Here's how the part is built. I have some questions about the finished solid (model axes, mm). Round coordinates to 2 decimals unless told otherwise and drop trailing zeros. Use one line per item in the form item = value. Start each with the question number.
Q1. I'm going to push flat-ended pins straight in: pin 1 Ø2 at (y, z) = (2, -63) entering from -X; pin 2 Ø1.2 at (y, z) = (2.5, 62) entering from -X. Where does each tip first touch, or does it pass through?
Q2. I need wall thicknesses on line 1 along Z through (x, y) = (-8.5, 0.95); line 2 along Z through (x, y) = (-76.5, 1.7); line 3 along X through (y, z) = (1.1, 21.5). Which ranges of each line are inside material? Lowest first, please. Write a range as from..to.
Q3. I want a section at A-A on y = 0.95. State how many separate pieces and enclosed holes the cut face has, and give its area (3 significant figures).
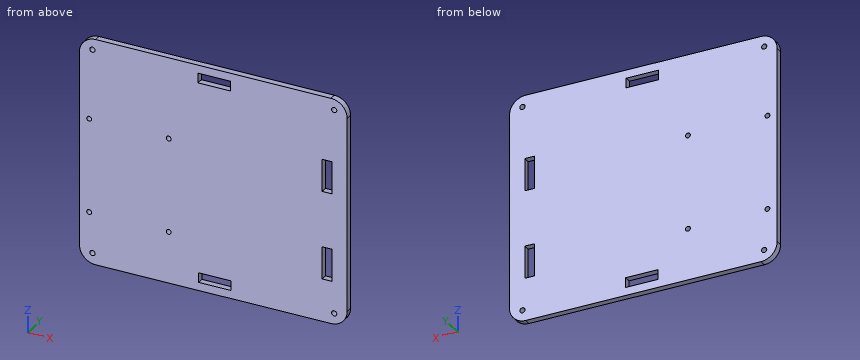
```python
from build123d import *

# Parameters (mm, degrees)
SKETCH1_W           = 165
SKETCH1_H           = 140
BOSS_EXTRUDE1_DEPTH = 4
SKETCH2_R           = 1.6
CUT_EXTRUDE1_DEPTH  = 10
FILLET1_R           = 10
SKETCH3_R           = 1.5
CUT_EXTRUDE2_DEPTH  = 10
SKETCH4_W           = 6
SKETCH4_H           = 20
SKETCH4_W_2         = 20
SKETCH4_H_2         = 6
CUT_EXTRUDE3_DEPTH  = 10


with BuildPart() as part:
    # Sketch1 → Boss-Extrude1 (new body)
    with BuildSketch(Plane(origin=(0, 0, 0), x_dir=(1, 0, 0), z_dir=(0, 1, 0))):
        Rectangle(SKETCH1_W, SKETCH1_H)
    extrude(amount=BOSS_EXTRUDE1_DEPTH)

    # Sketch2 → Cut-Extrude1 (cut)
    with BuildSketch(Plane(origin=(0, 4, 0), x_dir=(1, 0, 0), z_dir=(0, 1, 0))):
        with Locations(Location((-74.5, 63.212121212, 0), (0, 0, 270))):
            Circle(SKETCH2_R)
        with Locations(Location((-74.5, -63.212121212, 0), (0, 0, 270))):
            Circle(SKETCH2_R)
        with Locations(Location((74.5, -63.212121212, 0), (0, 0, 270))):
            Circle(SKETCH2_R)
        with Locations(Location((74.5, 63.212121212, 0), (0, 0, 270))):
            Circle(SKETCH2_R)
    extrude(amount=-CUT_EXTRUDE1_DEPTH, mode=Mode.SUBTRACT)

    # Fillet1
    fillet1_edges = [part.edges().sort_by_distance(p)[0] for p in [
        (82.5, 2, 70),
        (-82.5, 2, 70),
        (-82.5, 2, -70),
        (82.5, 2, -70),
    ]]
    fillet(fillet1_edges, radius=FILLET1_R)

    # Sketch3 → Cut-Extrude2 (cut)
    with BuildSketch(Plane(origin=(0, 4, 0), x_dir=(1, 0, 0), z_dir=(0, 1, 0))):
        with Locations(Location((-76.5, 38.189224362, 0), (0, 0, 270))):
            Circle(SKETCH3_R)
        with Locations(Location((-27.5, 38.189224362, 0), (0, 0, 270))):
            Circle(SKETCH3_R)
        with Locations(Location((-76.5, -19.810775638, 0), (0, 0, 270))):
            Circle(SKETCH3_R)
        with Locations(Location((-27.5, -19.810775638, 0), (0, 0, 270))):
            Circle(SKETCH3_R)
    extrude(amount=-CUT_EXTRUDE2_DEPTH, mode=Mode.SUBTRACT)

    # Sketch4 → Cut-Extrude3 (cut)
    with BuildSketch(Plane(origin=(0, 4, 0), x_dir=(1, 0, 0), z_dir=(0, 1, 0))):
        with Locations((70, 33.680953207)):
            Rectangle(SKETCH4_W, SKETCH4_H)
        with Locations((70, -20.735149517)):
            Rectangle(SKETCH4_W, SKETCH4_H)
        with Locations((0.550060732, -62)):
            Rectangle(SKETCH4_W_2, SKETCH4_H_2)
        with Locations((0.930649546, 62)):
            Rectangle(SKETCH4_W_2, SKETCH4_H_2)
    extrude(amount=-CUT_EXTRUDE3_DEPTH, mode=Mode.SUBTRACT)


solid = part.part
```
Reported:
q1.pin_1 = -82.3
q1.pin_2 = -82.4
q2.line_1 = -70..-65, -59..59, 65..70
q2.line_2 = -69.17..-39.69, -36.69..18.31, 21.31..69.17
q2.line_3 = -82.5..67, 73..82.5
q3.separate_pieces = 1
q3.enclosed_holes = 12
q3.area = 22,500 mm^2
